Here's how the part is built. I have some questions about the finished solid (model axes, mm). A direction names the side the tool comes from. Coordinates: 2 decimals unless noted, no trailing zeros. Write each loop counter-clockwise with the first axis right and the second up, starting at its lowest first coordinate (ties: lowest second). Pieces come first, ordered by that corner, then holes.
Item 1: I'm going to push flat-ended pins straight in: pin 1 Ø3 at (y, z) = (3, -4) entering from +X; pin 2 Ø12 at (x, z) = (5, 3) entering from +Y; pin 3 Ø2 at (y, z) = (6.5, -6) entering from +X. Where does each tip first touch, or does it pass through?
Item 2: If we section it at B-B (y = 8): Please give me the cut outline in (x, z), then the cut area to 3 significant figures.
Item 3: If we section it at A-A (x = 0): Please give me the cut outline in (y, z), then the cut area to 3 significant figures.
Item 4: If we section it at D-D (y = 1.5): Please give me the cut outline in (x, z).
Item 5: We'd pull the mould along Z, two halves only. Please class faces 1 (the face through (-13.67, 6.97, -3.03)), 2 (the face through (0, 2, 0)), 3 (the face through (0, 0, 0)): +Z half, -Z half, draft (parallel to the pull), parting line (faces both ways), or undercut.
Item 6: For faces 4 (the face through (-9.3, 9, 9.3)), 5 (the face through (-10, 6, 1)), which set-ups out of +Z, -Z, +X, -X, +Y, -Y let a thin tool reach every point of the face, with its end or its side?
Item 7: If I drill on line 1 (X direction, y = 7.45, z = 0); line 2 (Y direction, x = 1.5, z = -2.25); line 3 (X direction, y = 3.75, z = -7.25), over which ranges is the centre line in solid material (lowest first)?
Item 8: If we section it at C-C (z = 0): Please give me the cut outline in (x, y).
from build123d import *

# Parameters (mm, degrees)
ESQUISSE1_R             = 14
BOSS_EXTRU_1_DEPTH      = 9
ESQUISSE2_R             = 13
ENL_V_MAT_EXTRU_1_DEPTH = 3
ESQUISSE4_R             = 9.5
ENL_V_MAT_EXTRU_2_DEPTH = 4
CHANFREIN1_SIZE         = 5


with BuildPart() as part:
    # Esquisse1 → Boss.-Extru.1 (new body)
    with BuildSketch(Plane(origin=(0, 0, 0), x_dir=(1, 0, 0), z_dir=(0, 1, 0))):
        with Locations(Location((0, 0, 0), (0, 0, 270))):
            Circle(ESQUISSE1_R)
    extrude(amount=BOSS_EXTRU_1_DEPTH)

    # Esquisse2 → Enlèv. mat.-Extru.1 (cut)
    with BuildSketch(Plane(origin=(0, 9, 0), x_dir=(1, 0, 0), z_dir=(0, 1, 0))):
        with Locations(Location((0, 0, 0), (0, 0, 270))):
            Circle(ESQUISSE2_R)
    extrude(amount=-ENL_V_MAT_EXTRU_1_DEPTH, mode=Mode.SUBTRACT)

    # Esquisse4 → Enlèv. mat.-Extru.2 (cut)
    with BuildSketch(Plane(origin=(0, 6, 0), x_dir=(1, 0, 0), z_dir=(0, 1, 0))):
        with Locations(Location((0, 0, 0), (0, 0, 270))):
            Circle(ESQUISSE4_R)
    extrude(amount=-ENL_V_MAT_EXTRU_2_DEPTH, mode=Mode.SUBTRACT)

    # Chanfrein1
    chanfrein1_edges = [part.edges().sort_by_distance(p)[0] for p in [
        (0, 0, -14),
    ]]
    chamfer(chanfrein1_edges, length=CHANFREIN1_SIZE)


solid = part.part
Answer list:
1. pin 1: stops at x = 12.95
1. pin 2: stops at y = 6
1. pin 3: stops at x = 13.08
2. outline: circle Ø28 at (0, 0); hole circle Ø26 at (0, 0)
2. area: 84.8 mm2
3. outline: (0, -9) - (5, -14) - (9, -14) - (9, -13) - (6, -13) - (6, -9.5) - (2, -9.5) - (2, 9.5) - (6, 9.5) - (6, 13) - (9, 13) - (9, 14) - (5, 14) - (0, 9) - close
3. area: 73.0 mm2
4. outline: circle Ø21 at (0, 0)
5. face 1: parting line
5. face 2: undercut
5. face 3: draft
6. face 4: +Z, -Z, +X, -X, +Y
6. face 5: +Y
7. line 1: x = -14 to -13, 13 to 14
7. line 2: y = 0 to 2
7. line 3: x = -10.49 to -6.14, 6.14 to 10.49
8. outline: (-14, 5) - (-9, 0) - (9, 0) - (14, 5) - (14, 9) - (13, 9) - (13, 6) - (9.5, 6) - (9.5, 2) - (-9.5, 2) - (-9.5, 6) - (-13, 6) - (-13, 9) - (-14, 9) - close
